Autodesk Inventor part; units mm, degrees
ref_plane "YZ Plane" through (0, 0, 0) normal (1, 0, 0) x (0, 1, 0)
ref_plane "XZ Plane" through (0, 0, 0) normal (0, 1, 0) x (-1, 0, 0)
ref_plane "XY Plane" through (0, 0, 0) normal (0, 0, 1) x (1, 0, 0)
sketch "Skizze1" plane through (0, 0, 0) normal (0, 0, 1) x (1, 0, 0)
  circle A0 centre (0, 0) radius 22.5
  circle A1 centre (0, 0) radius 9
  dimension "d0" = 45
  dimension "d2" = 9
extrude "Extrusion1" add sketch "Skizze1" along normal blind 15
sketch "Skizze3" plane through (0, 0, 0) normal (0, 0, -1) x (-1, 0, 0)
  circle A0 centre (0, 0) radius 9
  circle A1 centre (0, 0) radius 22.5
  circle A2 centre (0, 0) radius 16
  dimension "d5" = 32
extrude "Extrusion2" cut sketch "Skizze3" against normal blind 8 contours A2
sketch "Skizze4" plane through (0, 0, 15) normal (0, 0, 1) x (1, 0, 0)
  circle A0 centre (0, 0) radius 9
  circle A1 centre (0, 0) radius 16
  line L0 (-27, 0) -> (36, 0)
  point P0 (-12.5, 0)
  point P1 (12.5, 0)
  dimension "d8" = 12.5
  dimension "d9" = 12.5
hole "Bohrung1" at (-12.5, 0, 15) at (12.5, 0, 15) direction (0, 0, -1) diameter 2 end through all countersink diameter 4 countersink angle 90
fillet "Rundung1" radius 1 2 edges at (-22.5, 0, 15) (-22.5, 0, 0)
properties part number "Griff01"
CAD build for the part. Positions are in the model's coordinates, mm. A direction names the side the tool comes from. Give positions to 0.01 mm unless a question says otherwise; leave off trailing zeros. Write each loop counter-clockwise with the first axis right and the second up, starting at its lowest first coordinate (ties: lowest second). Pieces come first, ordered by that corner, then holes. Notation, with made-up numbers: M 31,60 L 36,60 A16 ccw 36,89 Z; hole C 76,69 d5. An arc over 180 degrees is marked long. Put each result on its own line as item: value. Start each with the question number.
(1) Flat gauge pins, fed straight in: pin 1 Ø3 at (y, z) = (-9.5, 4) entering from -X; pin 2 Ø1.5 at (x, z) = (2, 7.5) entering from -Y; pin 3 Ø1.5 at (x, z) = (-10, 10) entering from -Y. Where does each tip first touch, or does it go through?
(2) Band-saw the part on A-A, the plane x = 0. Write the cut outline in (y, z), and give its area (3 significant figures).
(3) Which spindle directions (+Z, -Z, +X, -X, +Y, -Y) get a long thin tool onto all of the face, cutting with end or side? Do faces 5 (the face through (3.47, -15.62, 3.94)), 6 (the face through (13.39, -0.46, 10.96)). Say none if no direction does.
(4) Probe L1, parallel to Y at x = 0, z = 11.5; L2, parallel to X at y = 8, z = 3; L3, parallel to X at y = 3, z = 9.5. List the from-to ranges inside material, lowest first.
(5) Mould opens along Y. For faces 1 (the face through (-11.524, 0.217, 10.958)), 2 (the face through (10.382, 19.961, 7.409)), 3 (the face through (-0.3, -9.3, 15)), 4 (the face through (-1.172, -8.923, 11.451)) say: +Y half, -Y half, draft (parallel to the pull), parting line (faces both ways), or undercut.
(6) Band-saw the part on B-B, the plane z = 6.75. Write the cut outline in (x, y).
Response values:
1. pin 1: stops at x = -21.03
1. pin 2: stops at y = -22.47
1. pin 3: stops at y = -20.51
2. outline: M -22.5,1 A1 ccw -21.5,0 L -16,0 L -16,8 L -9,8 L -9,15 L -21.5,15 A1 ccw -22.5,14 Z; M 9,8 L 16,8 L 16,0 L 21.5,0 A1 ccw 22.5,1 L 22.5,14 A1 ccw 21.5,15 L 9,15 Z
2. area: 292 mm2
3. face 5: -Z
3. face 6: +Z, -Z
4. L1: y = -22.5 to -9, 9 to 22.5
4. L2: x = -21.03 to -13.86, 13.86 to 21.03
4. L3: x = -22.3 to -8.49, 8.49 to 22.3
5. face 1: undercut
5. face 2: parting line
5. face 3: draft
5. face 4: undercut
6. outline: C 0,0 d45; hole C 0,0 d32
